```python
from build123d import *

# Parameters (mm, degrees)
BOSS_EXTRUDE1_DEPTH             = 25.4
SKETCH2_R                       = 5.715
BOSS_EXTRUDE2_DEPTH             = 48.26
BOSS_EXTRUDE2_DIRECTION_2_REACH = 52.818
FILLET1_R                       = 1.27


with BuildPart() as part:
    # Sketch1 → Boss-Extrude1 (new body)
    with BuildSketch(Plane.XY):
        with BuildLine():
            ThreePointArc((-21.315601844, -20.824385658), (-19.601712639, -21.737702654), (-18.056418846, -20.5614241))
            add(Edge.make_bspline(
                [(2.526351365, 36.325614342), (-0.715696382, 5.186662468), (-18.056418846, -20.5614241)],
                knots=[0, 0, 0, 0.967613504, 0.967613504, 0.967613504], degree=2))
            ThreePointArc((2.526351365, 36.325614342), (1.317636804, 36.98031962), (0, 36.5885759))
            add(Edge.make_bspline(
                [(0, 36.5885759), (-3.282504286, 5.052562618), (-21.315601844, -20.824385658)],
                knots=[0, 0, 0, 1, 1, 1], degree=2))
        make_face()
    extrude(amount=BOSS_EXTRUDE1_DEPTH)

    # Sketch2 → Boss-Extrude2 (add)
    with BuildSketch(Plane(origin=(2.54, 0, 0), x_dir=(0, 0, -1), z_dir=(1, 0, 0))):
        with Locations((-12.812340203, 8.6485759)):
            Circle(SKETCH2_R)
    extrude(amount=BOSS_EXTRUDE2_DEPTH)

    # Sketch2 → Boss-Extrude2 direction 2 (add, up to next)
    with BuildSketch(Plane(origin=(2.54, 0, 0), x_dir=(0, 0, -1), z_dir=(1, 0, 0)), mode=Mode.PRIVATE) as boss_extrude2_direction_2_sk1:
        with Locations((-12.812340203, 8.6485759)):
            Circle(SKETCH2_R)
    boss_extrude2_direction_2_tool1 = extrude(boss_extrude2_direction_2_sk1.sketch, amount=-BOSS_EXTRUDE2_DIRECTION_2_REACH, mode=Mode.PRIVATE) - part.part
    add(boss_extrude2_direction_2_tool1.solids().sort_by_distance((2.54, 8.648576, 12.81234))[0])

    # Fillet1
    fillet1_edges = [part.edges().sort_by_distance(p)[0] for p in [
        (-6.955501037, 6.506813911, 25.4),
        (-6.955501037, 6.506813911, 0),
    ]]
    fillet(fillet1_edges, radius=FILLET1_R)


solid = part.part
```
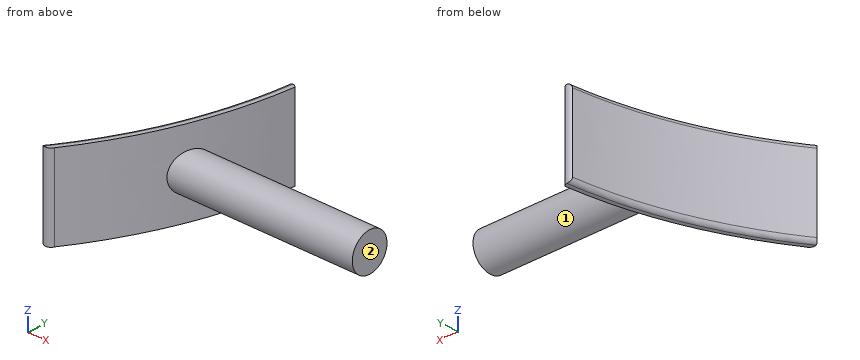
Geometry: final body of the model. Coordinates: model frame, mm. Face numbers are marked on the shaded views. A direction names the side the tool comes from. Coordinates: 2 decimals unless noted, no trailing zeros. Order: outer loops, then holes, each group sorted by start corner. A loop starts at its lowest first (then second) coordinate and runs counter-clockwise, first axis right, second up. Notation, with made-up numbers: (81.25, -28) - (120.25, -28) arc R19 cw to (120.25, 9) - close; hole circle Ø4 at (-40, 7.25). An arc over 180 degrees is marked (long way). Return JSON: item names as keys, results as strings. Group by question number.
1. Set-up query: the marked faces 1 and 2. Return all of +Z, -Z, +X, -X, +Y, -Y with unobstructed straight access to the full face (end or side cutting, diameter ignored); none if empty.
2. Cut plane A-A (x = 26). Output: boundary loops of the cut face in (y, z) (3 decimals).
3. Material intervals for line 1 along X through (y, z) = (28, 21.75); line 2 along X through (y, z) = (32, 12); line 3 along Y through (x, z) = (29.5, 13.5), sorted ascending. Write a range as [from, to].
4. Pin query (flat end, axial travel): pin 1 (12 mm diameter, centred on y = 29.5, z = 20, fed in from -X); pin 2 (6 mm diameter, centred on x = -3.5, z = 20.5, fed in from -Y); pin 3 (8 mm diameter, centred on x = 20.5, z = 21.5, fed in from +Y). Return the tip coordinate at first contact, or that it passes through.
Resolved:
{
 "1": {"face 1": "+X", "face 2": "+Z, -Z, +X, +Y, -Y"},
 "2": {"outline": "circle Ø11.43 at (8.649, 12.812)"},
 "3": {"line 1": "x = [-1.19, 1.39]", "line 2": "x = [-0.56, 2]", "line 3": "y = [2.98, 14.32]"},
 "4": {"pin 1": "stops at x = -2.05", "pin 2": "stops at y = 0.76", "pin 3": "stops at y = 11.92"}
}
